from build123d import *

# Parameters (mm, degrees)
SM_BASE_FLANGE_1_DEPTH = 50
SKETCH_2_R             = 6.5
CUT_EXTRUDE_1_DEPTH    = 10
CUT_EXTRUDE_2_DEPTH    = 10
SKETCH_4_R             = 6.5
CUT_EXTRUDE_3_DEPTH    = 10
SKETCH_5_R             = 6.5
CUT_EXTRUDE_4_DEPTH    = 10
OTHER_START            = -10
OTHER_1_DEPTH          = 10


# Read off the part's stored shape, not the designer's step: Затупленный угол1
# Sheet-metal steps are written as plain solids
with BuildPart() as part:
    # Sketch 1 → Базовая кромка1 (new body)
    with BuildSketch(Plane.XY):
        with BuildLine():
            Line((-381.414527052, -5), (-323.037303653, -5))
            ThreePointArc((-323.037303653, -5), (-321.435481223, -4.870874576), (-319.875025993, -4.486832981))
            Line((-319.875025993, -4.486832981), (-308.723778639, -0.769750529))
            ThreePointArc((-308.723778639, -0.769750529), (-306.383095794, -0.193688135), (-303.980362149, 0))
            Line((-303.980362149, 0), (468.585472948, 0))
            Line((468.585472948, 0), (468.585472948, -5))
            Line((468.585472948, -5), (-303.980362149, -5))
            ThreePointArc((-303.980362149, -5), (-305.582184579, -5.129125424), (-307.142639809, -5.513167019))
            Line((-307.142639809, -5.513167019), (-318.293887163, -9.230249471))
            ThreePointArc((-318.293887163, -9.230249471), (-320.634570008, -9.806311865), (-323.037303653, -10))
            Line((-323.037303653, -10), (-381.414527052, -10))
            Line((-381.414527052, -10), (-381.414527052, -5))
        make_face()
    extrude(amount=SM_BASE_FLANGE_1_DEPTH)

    # Sketch 2 → Вырез-Вытянуть1 (cut)
    with BuildSketch(Plane(origin=(0, 0, 0), x_dir=(1, 0, 0), z_dir=(0, 1, 0))):
        with Locations(Location((443.585472948, -25, 0), (0, 0, 270))):
            Circle(SKETCH_2_R)
    extrude(amount=-CUT_EXTRUDE_1_DEPTH, mode=Mode.SUBTRACT)

    # Эскиз3 → Вырез-Вытянуть2 (cut)
    with BuildSketch(Plane(origin=(0, 0, 0), x_dir=(1, 0, 0), z_dir=(0, 1, 0))):
        with BuildLine():
            Line((344.585472948, -18.5), (352.585472948, -18.5))
            ThreePointArc((352.585472948, -18.5), (359.085472948, -25), (352.585472948, -31.5))
            Line((352.585472948, -31.5), (344.585472948, -31.5))
            ThreePointArc((344.585472948, -31.5), (338.085472948, -25), (344.585472948, -18.5))
        make_face()
    extrude(amount=-CUT_EXTRUDE_2_DEPTH, mode=Mode.SUBTRACT)

    # Эскиз4 → Вырез-Вытянуть3 (cut)
    with BuildSketch(Plane(origin=(0, 0, 0), x_dir=(1, 0, 0), z_dir=(0, 1, 0))):
        with Locations(Location((120.585472948, -25, 0), (0, 0, 270))):
            Circle(SKETCH_4_R)
    extrude(amount=-CUT_EXTRUDE_3_DEPTH, mode=Mode.SUBTRACT)

    # Эскиз5 → Вырез-Вытянуть4 (cut)
    with BuildSketch(Plane(origin=(0, -5, 0), x_dir=(1, 0, 0), z_dir=(0, 1, 0))):
        with Locations(Location((-356.414527052, -25, 0), (0, 0, 270))):
            Circle(SKETCH_5_R)
    extrude(amount=-CUT_EXTRUDE_4_DEPTH, mode=Mode.SUBTRACT)

    # Other 1 outline → Other 1 (cut)
    with BuildSketch(Plane(origin=(0, 0, 0), x_dir=(1, 0, 0), z_dir=(0, 1, 0)).offset(OTHER_START)):
        Polygon((468.585472948, 0), (463.585472948, 0), (468.585472948, -5), align=None)
        Polygon((468.585472948, -50), (468.585472948, -45), (463.585472948, -50), align=None)
        Polygon((-381.414527052, 0), (-381.414527052, -5), (-376.414527052, 0), align=None)
        Polygon((-376.414527052, -50), (-381.414527052, -45), (-381.414527052, -50), align=None)
    extrude(amount=OTHER_1_DEPTH, mode=Mode.SUBTRACT)


solid = part.part
Design review of the part built by this model. Coordinates are the model's own, in mm. A direction names the side the tool comes from. Coordinates: 2 decimals unless noted, no trailing zeros. Loops run counter-clockwise (first coordinate to the right, second up) from the corner with the lowest first, then second, coordinate; pieces in that order, holes last. Notation, with made-up numbers: M 3.25,51 L 19.25,51 A29 ccw 19.25,82 Z; hole C 68.5,14.5 d9. An arc over 180 degrees is marked long. Use one line per item in the form item = value.
(1) Consider section B-B (x = 40.5). Write out the cut boundary in (y, z), and give its area (3 significant figures).
Return value:
outline = M -5,0 L 0,0 L 0,50 L -5,50 Z
area = 250 mm2
(2) For faces 4 (the face through (-362.76, -7.46, 23.59)), 5 (the face through (88, -5, 25)), list the 3-axis set-ups (+Z, -Z, +X, -X, +Y, -Y) from which the entire face can be reached by the end or side of a thin tool; tool diameter is ignored.
Return value:
face_4 = +Y, -Y
face_5 = +Z, -Z, +X, -Y
(3) Consider section A-A (y = -2.75). Write out the cut boundary in (x, z), and give its area (3 significant figures).
Return value:
outline = M -314.66,0 L 463.59,0 L 468.59,5 L 468.59,45 L 463.59,50 L -314.66,50 Z; hole C 120.59,25 d13; hole M 344.59,18.5 L 352.59,18.5 A6.5 ccw 352.59,31.5 L 344.59,31.5 A6.5 ccw Z; hole C 443.59,25 d13
area = 38,600 mm2
(4) Clearance check with flat-ended pins moving along their axes: P1, Ø25, axis at x = 47, z = 24.5, coming from the -Y side; P2, Ø1, axis at x = -246, y = -7, coming from the -Z side. State where each tip first meets the part, or that it passes through.
Return value:
P1 = -5
P2 = through
(5) Draft analysis for pull direction X (two halves, no side actions). For faces 1 (the face through (-353, -5, 19)), 2 (the face through (437.24, -2.46, 23.59)), 3 (the face through (120.871, -2.465, 18.506)), state which applies: pulls with the +X half, pulls with the -X half, needs draft (parallel to the pull), parting line crosses it, or undercut.
Return value:
face_1 = needs draft
face_2 = undercut
face_3 = undercut
(6) For line 1 along Y through (x, z) = (-46.5, 12); line 2 along Z through (x, y) = (118, -2.5), list the stretches that pass through material, from the lowest coordinate up. Write a range as from..to.
Return value:
line_1 = -5..0
line_2 = 0..19.04, 30.96..50
